Geometry: final body of the model. Coordinates: model frame, mm. A direction names the side the tool comes from. Coordinates: 2 decimals unless noted, no trailing zeros. Loops run counter-clockwise (first coordinate to the right, second up) from the corner with the lowest first, then second, coordinate; pieces in that order, holes last. Notation, with made-up numbers: (-22, 50) - (14, 50) arc R29 cw to (14, 74) - close; hole circle Ø7 at (12, 0.25). An arc over 180 degrees is marked (long way). Return JSON: item names as keys, results as strings.
from build123d import *

# Parameters (mm, degrees)
DOME2_FACE_RADIUS  = 3.302
DOME2_HEIGHT       = 2.54
CUT_EXTRUDE2_DEPTH = 21.698272827
SEEDCUT_COUNT      = 8


# Read off the part's stored shape, not the designer's step: Cut-Revolve-Thin5
with BuildPart() as part:
    # Sketch5 → Revolve1 (revolve)
    with BuildSketch(Plane(origin=(0, 0, 0), x_dir=(0, 0, -1), z_dir=(1, 0, 0)), mode=Mode.PRIVATE) as revolve1_sk:
        Polygon((-10.655580084, 0), (-10.655580084, 7.493), (-8.115580084, 7.493), (-8.115580084, 5.08), (4.584419916, 5.08), (4.584419916, 0), align=None)
    revolve(revolve1_sk.sketch.rotate(Axis((0, 0, 7.652463568), (0, 0, -1)), 90), axis=Axis((0, 0, 7.652463568), (0, 0, -1)))

    # Sketch8 → Revolve3 (revolve)
    with BuildSketch(Plane(origin=(0, 0, 0), x_dir=(0, 0, -1), z_dir=(1, 0, 0))):
        with BuildLine():
            Line((-20.257637537, 0), (-10.655580084, 0))
            Line((-10.655580084, 0), (-10.655580084, 6.146975902))
            add(Edge.make_bspline(
                [(-10.655580084, 6.146975902), (-14.696094585, 6.626842046), (-19.387675836, 4.389685938), (-20.257637537, 0)],
                knots=[0, 0, 0, 0, 1, 1, 1, 1], degree=3))
        make_face()
    revolve(axis=Axis((0, 0, 7.652463568), (0, 0, 1)))

    # Cut-Revolve-Thin5 outline → Cut-Revolve-Thin5 (revolve, cut)
    with BuildSketch(Plane.XZ):
        Polygon((3.302, -2.806419916), (3.302, -4.584419916), (5.08, -4.584419916), (5.08, 1.765580084), align=None)
    revolve(axis=Axis((0, 0, 0), (0, 0, 1)), mode=Mode.SUBTRACT)

    # Dome2: a dome of height H over a round flat face of radius A is a cap of a sphere of radius (A * A + H * H) / (2 * H)
    dome2_r = (DOME2_FACE_RADIUS * DOME2_FACE_RADIUS + DOME2_HEIGHT * DOME2_HEIGHT) / (2 * DOME2_HEIGHT)
    dome2_base = Plane((0, 0, -4.584419916), z_dir=(0, 0, -1))
    with Locations(dome2_base.offset(DOME2_HEIGHT - dome2_r)):
        dome2_ball = Sphere(dome2_r, mode=Mode.PRIVATE)
    add(split(dome2_ball, bisect_by=dome2_base, keep=Keep.TOP, mode=Mode.PRIVATE))

    # Sketch12 → Cut-Extrude2 (cut, through all)
    with BuildSketch(Plane.XY.offset(10.655580084)):
        with BuildLine():
            Line((0, 6.851966826), (0.615694723, 7.467661549))
            ThreePointArc((0.615694723, 7.467661549), (0, 7.493), (-0.615694723, 7.467661549))
            Line((-0.615694723, 7.467661549), (0, 6.851966826))
        make_face()
    cut_extrude2 = extrude(amount=-CUT_EXTRUDE2_DEPTH, mode=Mode.SUBTRACT)

    # SeedCut: Cut-Extrude2 ×8 about axis
    seedcut_axis = Axis((0, 0, 0), (0, 0, 1))
    for i in range(1, SEEDCUT_COUNT):
        add(cut_extrude2.rotate(seedcut_axis, i * 360 / SEEDCUT_COUNT), mode=Mode.SUBTRACT)


solid = part.part
Item 1: Section query A-A, the plane z = 9.5. Return loops of the section in (x, y).
Worked out:
{"outline": "(-7.47, -0.62) arc R7.49 ccw to (-5.72, -4.85) - (-4.85, -4.85) - (-4.85, -5.72) arc R7.49 ccw to (-0.62, -7.47) - (0, -6.85) - (0.62, -7.47) arc R7.49 ccw to (4.85, -5.72) - (4.85, -4.85) - (5.72, -4.85) arc R7.49 ccw to (7.47, -0.62) - (6.85, 0) - (7.47, 0.62) arc R7.49 ccw to (5.72, 4.85) - (4.85, 4.85) - (4.85, 5.72) arc R7.49 ccw to (0.62, 7.47) - (0, 6.85) - (-0.62, 7.47) arc R7.49 ccw to (-4.85, 5.72) - (-4.85, 4.85) - (-5.72, 4.85) arc R7.49 ccw to (-7.47, 0.62) - (-6.85, 0) - close"}
Item 2: Reachability of faces 1 (the face through (4.845, -5, 9)), 2 (the face through (-5, -4.845, 9)), 3 (the face through (5, 4.845, 9)), 4 (the face through (-5, 4.845, 9)) from +Z, -Z, +X, -X, +Y, -Y: full face, straight path, thin tool, end or side. Return the list, or none.
Worked out:
{"face 1": "+Z, -Z, +X, -Y", "face 2": "+Z, -Z, -X, -Y", "face 3": "+Z, -Z, +X, +Y", "face 4": "+Z, -Z, -X, +Y"}
Item 3: Section query B-B, the plane y = 6.5. Return loops of the section in (x, z).
Worked out:
{"outline": "(-3.73, 8.12) - (3.73, 8.12) - (3.73, 10.66) - (-3.73, 10.66) - close"}
Item 4: First-contact query: pin 1 Ø5 at (y, z) = (-0.5, 14.5) entering from -X; pin 2 Ø2 at (y, z) = (4.5, 12) entering from -X; pin 3 Ø0.7 at (y, z) = (5.5, 9.5) entering from -X; pin 4 Ø8 at (x, z) = (-2.5, 5.5) entering from +Y. Flat tips, straight axial feed; report the tip coordinate or a pass-through.
Worked out:
{"pin 1": "x = -6.21", "pin 2": "x = -5.13", "pin 3": "x = -4.85", "pin 4": "y = 7.47"}
Item 5: Ray query, probe 1 along Z at (x, y) = (-6, -2); probe 2 along X at (y, z) = (2.25, 16.25); probe 3 along X at (y, z) = (-0.75, 12.5). Return the intervals inside material, ascending. Write a range as from..to.
Worked out:
{"probe 1": "8.12..10.66", "probe 2": "-4.6..4.6", "probe 3": "-6.14..6.14"}
Item 6: Section query C-C, the plane z = -1.5. Return loops of the section in (x, y), and give its area (3 significant figures).
Worked out:
{"outline": "circle Ø7.62 at (0, 0)", "area": "45.6 mm^2"}
